Here's the drawing with two shaded views (mm, measured from the low corner). I have some questions. A direction names the side the tool comes from. Give positions to 0.01 mm unless a question says otherwise; leave off trailing zeros. Write each loop counter-clockwise with the first axis right and the second up, starting at its lowest first coordinate (ties: lowest second). Pieces come first, ordered by that corner, then holes. Notation, with made-up numbers: M 28.5,9 L 51.5,9 A9 ccw 51.5,14 Z; hole C -19.5,-11 d10. An arc over 180 degrees is marked long. Answer as CSV lines item,"result". Start each with the question number.
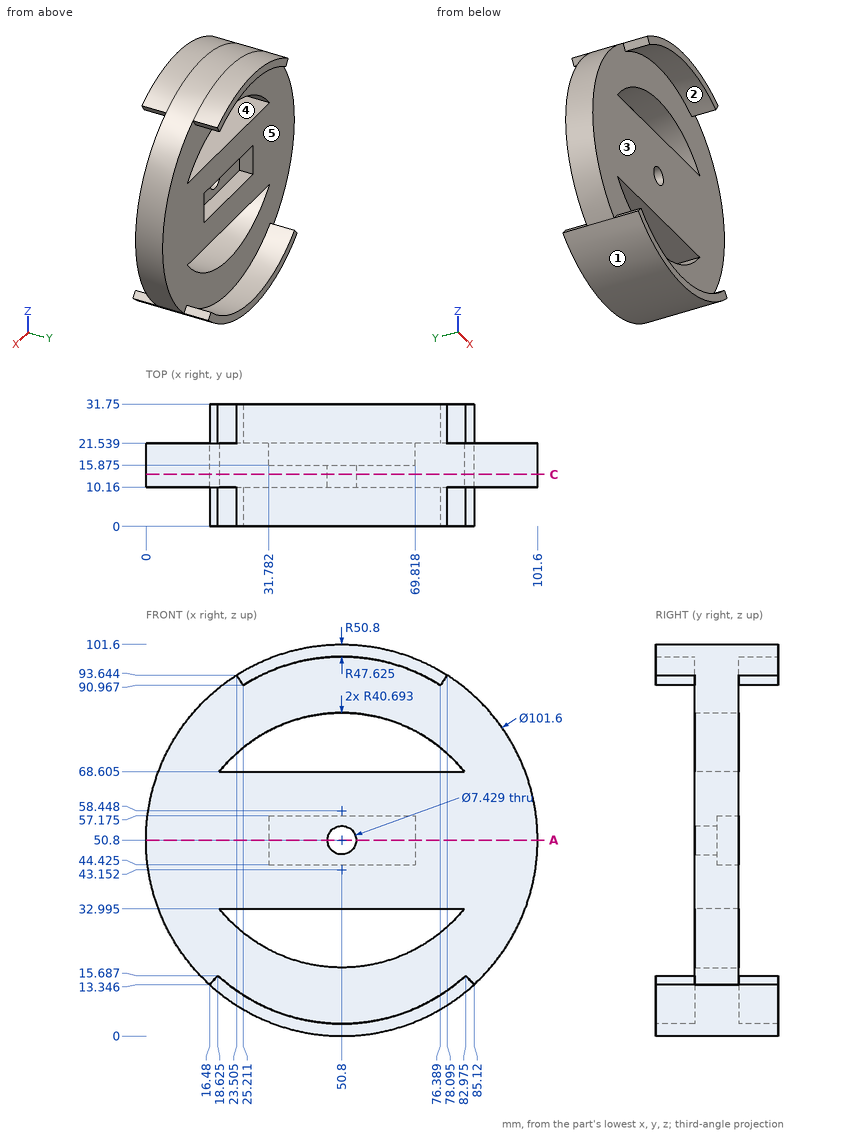
1. Will these pins go through, and if not, where does the flat tip stop? P1, Ø3.5, axis at x = 39, y = 13, coming from the +Z side; P2, Ø1.5, axis at y = 22.5, z = 90.5, coming from the +X side; P3, Ø14, axis at x = 49.5, z = 52.5, coming from the +Y side.
2. On a 3-axis mill with a long thin cutter (end or side, diameter ignored), from which of +Z, -Z, +X, -X, +Y, -Y can I reach the whole of each face in a straight line? I mean the marked faces 3, 4 and 5. Say none if no direction works.
3. Thinking about a two-plate mould opening in Z: for the marked faces 1 and 2, which applies, pulls with the +Z half, pulls with the -Z half, needs draft (parallel to the pull), parting line crosses it, or undercut?
4. Imagine slicing it at A-A, the plane z = 50.8. Please give me the cut outline in (x, y) (1 decimal).
5. Please list where these lines run through material, in increasing order: line 1 (Z direction, x = 50.8, y = 11.9) (1 decimal); line 2 (X direction, y = 11.85, z = 50.8) (1 decimal); line 3 (Z direction, x = 50.5, y = 6) (1 decimal).
6. Imagine slicing it at C-C, the plane y = 13.5. State how many separate pieces and enclosed holes the cut face has, plus the area to 3 significant figures.
Solutions:
1,P1,"z = 100.6"
1,P2,"x = 76.57"
1,P3,"y = 21.54"
2,face 3,"-Y"
2,face 4,"+Y, -Y"
2,face 5,"+Y"
3,face 1,"pulls with the -Z half"
3,face 2,"undercut"
4,outline,"M 0,10.2 L 47.1,10.2 L 47.1,15.9 L 31.8,15.9 L 31.8,21.5 L 0,21.5 Z; M 54.5,10.2 L 101.6,10.2 L 101.6,21.5 L 69.8,21.5 L 69.8,15.9 L 54.5,15.9 Z"
5,line 1,"0 to 17.8, 33 to 47.1, 54.5 to 68.6, 83.8 to 101.6"
5,line 2,"0 to 47.1, 54.5 to 101.6"
5,line 3,"0 to 3.2, 98.4 to 101.6"
6,separate pieces,"1"
6,enclosed holes,"3"
6,area,"6,720 mm²"
